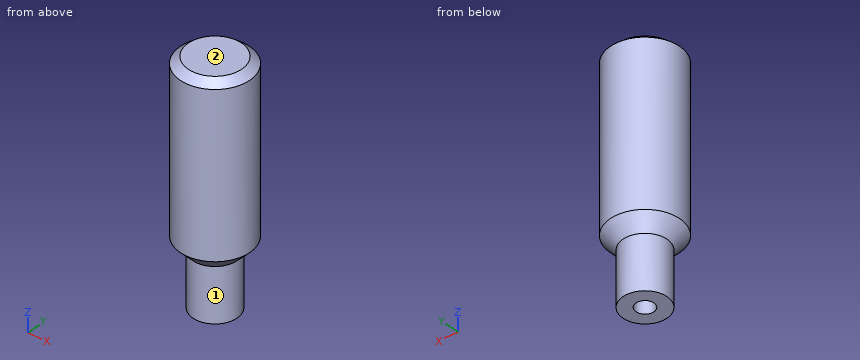
```python
from build123d import *

# Parameters (mm, degrees)
F0_R     = 16.5
F0_R_2   = 6.75
F1_DEPTH = 40
F4_R     = 26
F5_DEPTH = 120


with BuildPart() as f1:
    # F0 (on Top) → F1 (new body)
    with BuildSketch(Plane.XY):
        Circle(F0_R)
        Circle(F0_R_2, mode=Mode.SUBTRACT)
    extrude(amount=F1_DEPTH)

    # F2 (on Front) → F3 (revolve)
    with BuildSketch(Plane.XZ):
        Polygon((0, 39.999226), (16.5, 39.999226), (26, 49.999226), (0, 49.999226), align=None)
    revolve(axis=Axis((0, 0, 44.999226), (0, 0, 1)))

    # F4 (on face) → F5 (join)
    with BuildSketch(Plane.XY.offset(49.999226)):
        Circle(F4_R)
    extrude(amount=F5_DEPTH)

    # F6 (on Front) → F7 (revolve)
    with BuildSketch(Plane.XZ):
        Polygon((0, 169.999226), (0, 174.999226), (-20, 174.999226), (-26, 169.999226), align=None)
    revolve(axis=Axis((0, 0, 172.499226), (0, 0, 1)))


solid = f1.part
```
Verification items for the finished model (mm, model axes). Face numbers are marked on the shaded views. A direction names the side the tool comes from. Coordinates: 2 decimals unless noted, no trailing zeros. Write each loop counter-clockwise with the first axis right and the second up, starting at its lowest first coordinate (ties: lowest second). Pieces come first, ordered by that corner, then holes. Notation, with made-up numbers: (32.25, 46) - (39.25, 46) arc R30 ccw to (39.25, 80) - close; hole circle Ø11 at (-19.75, 33.25). An arc over 180 degrees is marked (long way). Write item = value, one per line.
Q1. Cross-section at A-A (y = 0). Enter the section's corners in (x, z).
Answer:
outline = (-26, 50) - (-16.5, 40) - (-16.5, 0) - (-6.75, 0) - (-6.75, 40) - (6.75, 40) - (6.75, 0) - (16.5, 0) - (16.5, 40) - (26, 50) - (26, 170) - (20, 175) - (-20, 175) - (-26, 170) - close
Q2. Access from +Z, -Z, +X, -X, +Y, -Y to the whole of each face (thin tool, end or side, straight path). Record for the marked faces 1 and 2.
Answer:
face_1 = -Z
face_2 = +Z, +X, -X, +Y, -Y
Q3. Cross-section at C-C (z = 23). Enter the section's corners in (x, y).
Answer:
outline = circle Ø33 at (0, 0); hole circle Ø13.5 at (0, 0)
Q4. Go/stop test with flat-tipped pins: pin 1 Ø3 at (x, y) = (14.5, -11) entering from -Z; pin 2 Ø1.5 at (y, z) = (19.5, 106.5) entering from +X; pin 3 Ø1.5 at (x, z) = (20, 70.5) entering from -Y. Record where each tip stops, or that it passes through.
Answer:
pin_1 = 40.21
pin_2 = 18.01
pin_3 = -17.48
Q5. Material ranges on L1, parallel to Y at x = 0, z = 28; L2, parallel to Y at x = -21, z = 68; L3, parallel to X at y = 23, z = 66, recorded low to high. Write a range as from..to.
Answer:
L1 = -16.5..-6.75, 6.75..16.5
L2 = -15.33..15.33
L3 = -12.12..12.12
Q6. Cross-section at D-D (z = 97.5). Enter the section's corners in (x, y).
Answer:
outline = circle Ø52 at (0, 0)
